```python
from build123d import *

# Parameters (mm, degrees)
SKETCH_1_R          = 12
EXTRUDE_1_DEPTH     = 2
SKETCH_2_R          = 10
EXTRUDE_2_DEPTH     = 10
SKETCH_3_R          = 0.75
CUT_EXTRUDE_1_DEPTH = 30


with BuildPart() as part:
    # 草图1 → 凸台-拉伸1 (new body)
    with BuildSketch(Plane(origin=(0, 0, 0), x_dir=(1, 0, 0), z_dir=(0, 1, 0))):
        with Locations(Location((0, 0, 0), (0, 0, 270))):
            Circle(SKETCH_1_R)
    extrude(amount=EXTRUDE_1_DEPTH)

    # 草图2 → 凸台-拉伸2 (add)
    with BuildSketch(Plane(origin=(0, 2, 0), x_dir=(1, 0, 0), z_dir=(0, 1, 0))):
        with Locations(Location((0, 0, 0), (0, 0, 270))):
            Circle(SKETCH_2_R)
    extrude(amount=EXTRUDE_2_DEPTH)

    # 草图3 → 切除-拉伸1 (cut, symmetric)
    with BuildSketch(Plane.XY):
        with Locations((0, 7)):
            Circle(SKETCH_3_R)
    extrude(amount=CUT_EXTRUDE_1_DEPTH, both=True, mode=Mode.SUBTRACT)


solid = part.part
```
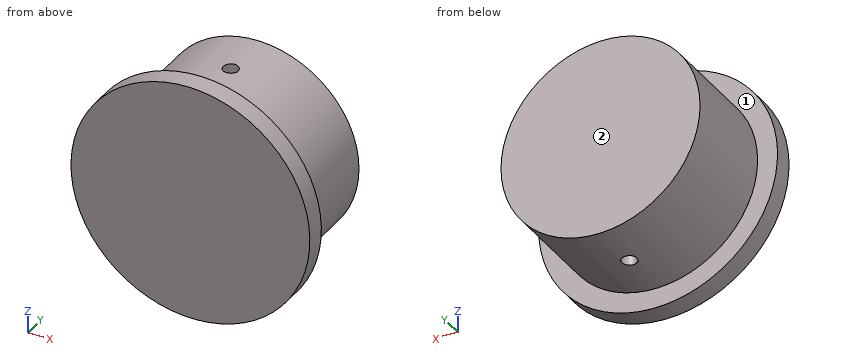
Here's how the part is built. I have some questions about the finished solid (model axes, mm). Face numbers are marked on the shaded views. A direction names the side the tool comes from. Coordinates: 2 decimals unless noted, no trailing zeros. Order: outer loops, then holes, each group sorted by start corner. A loop starts at its lowest first (then second) coordinate and runs counter-clockwise, first axis right, second up. Notation, with made-up numbers: (31.5, 15.5) -> (72.5, 15.5) arc R24 cw to (72.5, 38.5) -> close; hole circle Ø2 at (53.5, -0.75). An arc over 180 degrees is marked (long way). Return JSON: item names as keys, results as strings.
1) On a 3-axis mill with a long thin cutter (end or side, diameter ignored), from which of +Z, -Z, +X, -X, +Y, -Y can I reach the whole of each face in a straight line? I mean the marked faces 1 and 2. Say none if no direction works.
Conclusion:
{"face 1": "+Y", "face 2": "+Z, -Z, +X, -X, +Y"}
2) If I drill on probe 1 along Y at (x, z) = (0, -4); probe 2 along X at (y, z) = (7, 0.25); probe 3 along X at (y, z) = (7, 5.25), over which ranges is the centre line in solid material (lowest first)?
Conclusion:
{"probe 1": "y = 0 to 6.25, 7.75 to 12", "probe 2": "x = -10 to -0.75, 0.75 to 10", "probe 3": "x = -8.51 to -0.75, 0.75 to 8.51"}
3) If we section it at A-A on z = 0: List the corners of the cut face in (x, y) for me, plus the area to 3 significant figures.
Conclusion:
{"outline": "(-12, 0) -> (12, 0) -> (12, 2) -> (10, 2) -> (10, 12) -> (-10, 12) -> (-10, 2) -> (-12, 2) -> close; hole circle Ø1.5 at (0, 7)", "area": "246 mm²"}
4) If we section it at C-C on x = 4.25: List the corners of the cut face in (y, z) for me.
Conclusion:
{"outline": "(0, -11.22) -> (2, -11.22) -> (2, -9.05) -> (12, -9.05) -> (12, 9.05) -> (2, 9.05) -> (2, 11.22) -> (0, 11.22) -> close"}
5) If we section it at D-D on y = 9.75: List the corners of the cut face in (x, z) for me.
Conclusion:
{"outline": "circle Ø20 at (0, 0)"}
6) If we section it at B-B on x = 0: List the corners of the cut face in (y, z) for me.
Conclusion:
{"outline": "(0, -12) -> (2, -12) -> (2, -10) -> (6.25, -10) -> (6.25, 10) -> (2, 10) -> (2, 12) -> (0, 12) -> close; (7.75, -10) -> (12, -10) -> (12, 10) -> (7.75, 10) -> close"}
7) I'm going to push flat-ended pins straight in: P1, Ø3, axis at x = 4, y = 7, coming from the +Z side; P2, Ø1.5, axis at y = 5, z = 1.5, coming from the -X side; P3, Ø5, axis at x = 7, y = 3, coming from the -Z side. Where does each tip first touch, or does it pass through?
Conclusion:
{"P1": "stops at z = 9.68", "P2": "stops at x = -9.97", "P3": "stops at z = -11.04"}
